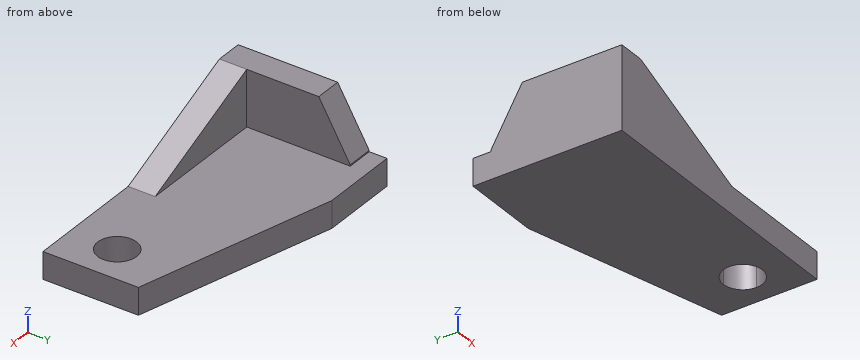
```python
from build123d import *

# Parameters (mm, degrees)
F1_DEPTH   = 10.922
F2_DEPTH   = 33.528
F2_FACE1_W = 10.922
F2_FACE1_H = 22.606
F4_DEPTH   = 53.594
F5_SIZE2   = 12.7582862486
F5_SIZE    = 22.098


with BuildPart() as f1:
    # F0 (on Top) → F1 (new body)
    with BuildSketch(Plane.XY):
        Polygon((-15.4502129098, 28.784671135), (-47.2277541757, 28.784671135), (-47.2277541757, 21.5939618647), (-36.3057541757, 21.5939618647), (-36.4225804595, -20.345826518), (16.1552155546, -20.4922857339), (16.2997870902, -31.413328865), (65.234824773, -31.413328865), (65.234824773, 7.1651804467), align=None)
        with BuildLine():
            ThreePointArc((49.9557780186, -4.2500742092), (55.5235368137, -6.5563154141), (57.8297780186, -12.1240742092))
            ThreePointArc((57.8297780186, -12.1240742092), (44.3880192235, -17.6918330042), (49.9557780186, -4.2500742092))
        make_face(mode=Mode.SUBTRACT)
    extrude(amount=F1_DEPTH)

    # F0 (on Top) → F2 (join)
    with BuildSketch(Plane.XY):
        Polygon((-36.3057541757, 21.5939618647), (-47.2277541757, 21.5939618647), (-47.2277541757, -31.413328865), (-36.4534097798, -31.413328865), (-36.4225804595, -20.345826518), align=None)
        Polygon((-36.4225804595, -20.345826518), (-36.4534097798, -31.413328865), (-15.4502129098, -31.413328865), (16.2997870902, -31.413328865), (16.1552155546, -20.4922857339), align=None)
    extrude(amount=F2_DEPTH)

    # F3 (on face) + F2_face1 (on face) → F4 (cut)
    with BuildSketch(Plane(origin=(-0.0569569325, -20.4471255665, 0), x_dir=(-0.9999961203, 0.0027855608, 0), z_dir=(0.0027855608, 0.9999961203, 0))):
        Polygon((-16.2122353854, 10.922), (36.3657646146, 33.528), (-16.2122353854, 33.528), align=None)
    with BuildSketch(Plane(origin=(16.2275013224, -25.9528072994, 22.225), x_dir=(-0.0132367273, 0.9999123907, 0), z_dir=(0.9999123907, 0.0132367273, 0))):
        Rectangle(F2_FACE1_W, F2_FACE1_H)
    extrude(amount=-F4_DEPTH, dir=(0.0027855608, 0.9999961203, 0), mode=Mode.SUBTRACT)

    # F5
    f5_edges = [f1.edges().sort_by_distance(p)[0] for p in [
        (-41.766754, 21.593962, 33.528),
    ]]
    f5_side = f1.faces().sort_by_distance((-41.766754, 21.593962, 22.225))[0]
    chamfer(f5_edges, length=F5_SIZE, length2=F5_SIZE2, reference=f5_side)


solid = f1.part
```
Check sheet for the modelled part. Datum: model origin and axes. Units: mm. Give positions to 0.01 mm unless a question says otherwise; leave off trailing zeros. Loops run counter-clockwise (first coordinate to the right, second up) from the corner with the lowest first, then second, coordinate; pieces in that order, holes last. Notation, with made-up numbers: (61.25, 17.5) - (112.25, 17.5) arc R21 ccw to (112.25, 48.5) - close; hole circle Ø6 at (32.5, 82.5). An arc over 180 degrees is marked (long way). One line per question, with ' | ' between items. Start each with the question number.
1. Gauge pin test, flat ends, axial feed: pin 1 Ø5 at (x, y) = (48.5, 4) entering from -Z; pin 2 Ø8 at (x, y) = (40.5, -12.5) entering from +Z; pin 3 Ø10 at (x, y) = (20.5, -23) entering from +Z; pin 4 Ø10 at (x, z) = (38.5, 19) entering from +Y. Record the tip position at first contact, or that the pin passes through.
2. Material ranges on line 1 along X through (y, z) = (6, 19); line 2 along Z through (x, y) = (-8, 10); line 3 along Y through (x, z) = (-35.5, 17.5), recorded low to high. Write a range as [from, to].
3. Cross-section at B-B, the plane y = -10. Enter the section's corners in (x, z), plus the area to 3 significant figures.
4. Cross-section at A-A, the plane z = 6. Enter the section's corners in (x, y), plus the area to 3 significant figures.
5. Cross-section at D-D, the plane y = -24. Enter the section's corners in (x, z).
6. Cross-section at C-C, the plane x = 56. Enter the section's corners in (y, z), plus the area to 3 significant figures.
Check result:
1) pin 1: stops at z = 0 | pin 2: stops at z = 10.92 | pin 3: stops at z = 11.2 | pin 4: passes through
2) line 1: x = [-47.23, -36.35] | line 2: z = [0, 10.92] | line 3: y = [-31.41, -20.35]
3) outline: (-47.23, 0) - (42.37, 0) - (42.37, 10.92) - (-36.39, 10.92) - (-36.39, 33.53) - (-47.23, 33.53) - close; (57.54, 0) - (65.23, 0) - (65.23, 10.92) - (57.54, 10.92) - close | area: 1,310 mm2
4) outline: (-47.23, -31.41) - (65.23, -31.41) - (65.23, 7.17) - (-15.45, 28.78) - (-47.23, 28.78) - close; hole circle Ø15.75 at (49.96, -12.12) | area: 5,700 mm2
5) outline: (-47.23, 0) - (65.23, 0) - (65.23, 10.92) - (16.15, 10.92) - (-36.43, 33.53) - (-47.23, 33.53) - close
6) outline: (-31.41, 0) - (-17.17, 0) - (-17.17, 10.92) - (-31.41, 10.92) - close; (-7.08, 0) - (9.64, 0) - (9.64, 10.92) - (-7.08, 10.92) - close | area: 338 mm2
